Autodesk Inventor part; units mm, degrees
ref_plane "YZ Plane" through (0, 0, 0) normal (1, 0, 0) x (0, 1, 0)
ref_plane "XZ Plane" through (0, 0, 0) normal (0, 1, 0) x (-1, 0, 0)
ref_plane "XY Plane" through (0, 0, 0) normal (0, 0, 1) x (1, 0, 0)
sketch "Sketch1" plane through (0, 0, 0) normal (0, 1, 0) x (-1, 0, 0)
  line L0 (0, 0) -> (25.4, 0)
  line L1 (25.4, 0) -> (25.4, 23.8125)
  line L2 (25.4, 23.8125) -> (0, 23.8125)
  line L3 (0, 23.8125) -> (0, 0)
  circle A0 centre (12.7, 11.1125) radius 6.35
  line L4 (12.7, 23.8125) -> (12.7, 0) construction
  line L5 (-19.05, 6.35) -> (-19.05, 0)
  line L6 (-19.05, 0) -> (0, 0)
  line L7 (44.45, 6.35) -> (44.45, 0)
  line L8 (44.45, 0) -> (25.4, 0)
  line L9 (-19.05, 6.35) -> (0, 6.35)
  line L10 (25.4, 6.35) -> (44.45, 6.35)
  dimension "d0" = 25.4
  dimension "d1" = 23.8125
  dimension "d2" = 12.7
  dimension "d9" = 6.35
  dimension "d10" = 19.05
  dimension "d11" = 19.05
  dimension "d12" = 6.35
  dimension "d20" = 11.1125
extrude "Extrusion1" add sketch "Sketch1" along normal blind 25.4
fillet "Fillet1" radius 12.7 2 edges at (-25.4, 12.7, 23.8125) (0, 12.7, 23.8125)
fillet "Fillet1" radius 1.5875 4 edges at (-25.4, 12.7, 6.35) (0, 12.7, 6.35) (-44.45, 12.7, 6.35) (19.05, 12.7, 6.35)
sketch "Sketch2" plane through (19.05, 25.4, 0) normal (0, 0, -1) x (-1, 0, 0)
  line L0 (1.5875, 0) -> (1.5875, -25.4) construction
  line L1 (17.4625, 0) -> (1.5875, 0) construction
  line L2 (17.4625, -25.4) -> (17.4625, 0) construction
  line L3 (61.9125, -25.4) -> (61.9125, 0) construction
  line L4 (46.0375, 0) -> (46.0375, -25.4) construction
  line L5 (61.9125, 0) -> (46.0375, 0) construction
  line L6 (1.5875, -12.7) -> (17.4625, -12.7) construction
  line L7 (46.0375, -12.7) -> (61.9125, -12.7) construction
  circle A0 centre (9.525, -12.7) radius 3.302
  circle A1 centre (53.975, -12.7) radius 3.302
  line L8 (61.9125, -25.4) -> (46.0375, -25.4)
  line L9 (17.4625, -25.4) -> (1.5875, -25.4)
  point P0 (19.05, -25.4)
  dimension "d15" = 6.604
  dimension "d16" = 6.604
  dimension "d21" = 44.45
extrude "Extrusion3" cut sketch "Sketch2" against normal through all
equation "\"d9\" = d12"
equation "\"d10\" = d11"
equation "\"d16\" = d15"
properties part number "Shaft Mount V1.500 Drivetrain" material "Aluminum 6061"
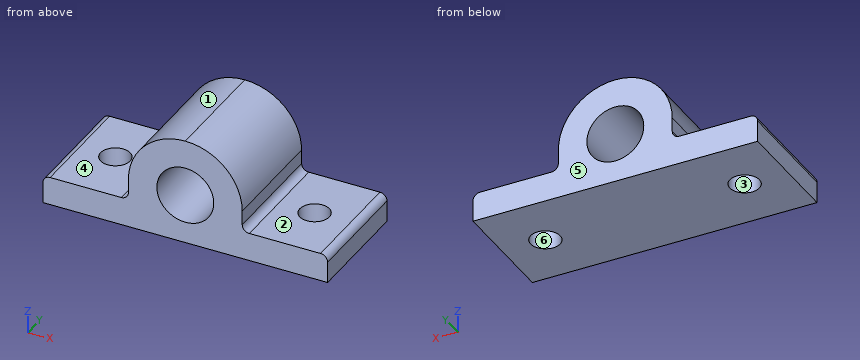
For this review, take the finished solid that the model builds, in its own axes (mm). Face numbers are marked on the shaded views. A direction names the side the tool comes from. Round coordinates to 2 decimals unless told otherwise and drop trailing zeros. Write each loop counter-clockwise with the first axis right and the second up, starting at its lowest first coordinate (ties: lowest second). Pieces come first, ordered by that corner, then holes. Notation, with made-up numbers: (75, -30.5) -> (83, -30.5) arc R18 cw to (83, 3.5) -> close; hole circle Ø5 at (-33.5, 11.5). An arc over 180 degrees is marked (long way). One line per question, with ' | ' between items. Start each with the question number.
1) For pin 1 Ø2 at (x, y) = (-17.5, 19.5) entering from -Z; pin 2 Ø5.5 at (x, y) = (-34.925, 12.7) entering from -Z; pin 3 Ø1.6 at (y, z) = (9, 9) entering from -X; pin 4 Ø12.5 at (x, y) = (-36.5, 12.5) entering from +Z, all flat-tipped, find the tip position at first contact; note any pin that passes through.
2) Add section B-B (x = -8.5). Write out the cut boundary in (y, z).
3) Machinability: for the marked faces 1 and 2, which of the approach directions +Z, -Z, +X, -X, +Y, -Y give a long, thin tool a straight path to every point of the face, cutting with its end or side? Answer none if there is none.
4) Add section C-C (z = 16.75). Write out the cut boundary in (x, y), and give its area (3 significant figures).
5) Wall thickness on line 1 along X through (y, z) = (11.5, 4.25); line 2 along Z through (x, y) = (-12.7, 6); line 3 along Z through (x, y) = (-28, 22.5): over which ranges is each line inside the solid? List them lowest first.
6) Mouldability with a two-part tool opening along Y and no side actions: class the marked faces 3, 4, 5 and 6 as +Y half, -Y half, draft (parallel to the pull), parting line (faces both ways), or undercut.
7) Add section A-A (y = 12.7). Count the separate pieces of the cut face and the enclosed holes in it, and give its area (3 significant figures).
Reported:
1) pin 1: stops at z = 0 | pin 2: passes through | pin 3: stops at x = -25.4 | pin 4: stops at z = 6.35
2) outline: (0, 0) -> (25.4, 0) -> (25.4, 6.35) -> (0, 6.35) -> close; (0, 15.88) -> (25.4, 15.88) -> (25.4, 23.1) -> (0, 23.1) -> close
3) face 1: +Z, -X, +Y, -Y | face 2: +Z, +X, +Y, -Y
4) outline: (-24.08, 0) -> (-15.62, 0) -> (-15.62, 25.4) -> (-24.08, 25.4) -> close; (-9.78, 0) -> (-1.32, 0) -> (-1.32, 25.4) -> (-9.78, 25.4) -> close | area: 430 mm²
5) line 1: x = -44.45 to -38, -31.85 to 6.45, 12.6 to 19.05 | line 2: z = 0 to 4.76, 17.46 to 23.81 | line 3: z = 0 to 6.35
6) face 3: undercut | face 4: draft | face 5: +Y half | face 6: undercut
7) separate pieces: 3 | enclosed holes: 1 | area: 567 mm²
